Work out the finished part from the listing and answer in its coordinate system (mm). Face numbers are marked on the shaded views. A direction names the side the tool comes from. Give positions to 0.01 mm unless a question says otherwise; leave off trailing zeros. Write each loop counter-clockwise with the first axis right and the second up, starting at its lowest first coordinate (ties: lowest second). Pieces come first, ordered by that corner, then holes. Notation, with made-up numbers: (-24.75, 26) - (-9.75, 26) arc R23 ccw to (-9.75, 36) - close; hole circle Ø10 at (13, 31.25). An arc over 180 degrees is marked (long way). Write item = value, one per line.
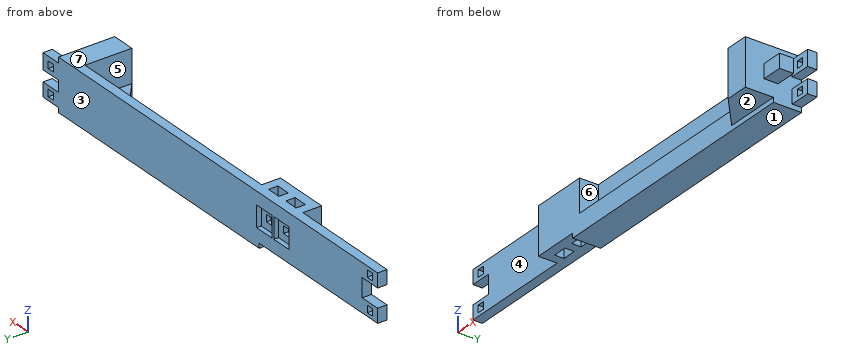
from build123d import *

# Parameters (mm, degrees)
SKETCH2_W           = 194.96
SKETCH2_H           = 6
BOSS_EXTRUDE1_DEPTH = 4
SKETCH3_W           = 176.96
SKETCH3_H           = 4
BOSS_EXTRUDE2_DEPTH = 14
SKETCH4_W           = 6
SKETCH4_H           = 4
BOSS_EXTRUDE3_DEPTH = 9
SKETCH5_W           = 6.8
SKETCH5_H           = 4
BOSS_EXTRUDE4_DEPTH = 9
CUT_EXTRUDE1_REACH  = 197.503
SKETCH6_W           = 3
SKETCH6_H           = 3
SKETCH7_W           = 10
SKETCH7_H           = 20
BOSS_EXTRUDE5_DEPTH = 20
SKETCH8_W           = 136.96
SKETCH8_H           = 6
BOSS_EXTRUDE6_DEPTH = 8
CHAMFER1_SIZE2      = 14.301043111
CHAMFER1_SIZE       = 12
BOSS_EXTRUDE7_DEPTH = 14
CUT_EXTRUDE2_REACH  = 199.001
SKETCH10_W          = 6
SKETCH10_H          = 4
CUT_EXTRUDE3_REACH  = 198.93
SKETCH11_W          = 3
SKETCH11_H          = 3
SKETCH12_W          = 116.96
SKETCH12_H          = 12
BOSS_EXTRUDE8_DEPTH = 2
SKETCH13_W          = 6
SKETCH13_H          = 6
BOSS_EXTRUDE9_DEPTH = 9
SKETCH14_W          = 9
SKETCH14_H          = 9
CUT_EXTRUDE4_DEPTH  = 2


with BuildPart() as part:
    # Sketch2 → Boss-Extrude1 (new body)
    with BuildSketch(Plane(origin=(0, 0, 0), x_dir=(1, 0, 0), z_dir=(0, 1, 0))):
        with Locations((97.48, 3)):
            Rectangle(SKETCH2_W, SKETCH2_H)
    extrude(amount=BOSS_EXTRUDE1_DEPTH)

    # Sketch3 → Boss-Extrude2 (add)
    with BuildSketch(Plane(origin=(0, 0, 0), x_dir=(-1, 0, 0), z_dir=(0, 0, -1))):
        with Locations((-97.48, 2)):
            Rectangle(SKETCH3_W, SKETCH3_H)
    extrude(amount=-BOSS_EXTRUDE2_DEPTH)

    # Sketch4 → Boss-Extrude3 (add)
    with BuildSketch(Plane.ZY.offset(-9)):
        with Locations((11, 2)):
            Rectangle(SKETCH4_W, SKETCH4_H)
    extrude(amount=BOSS_EXTRUDE3_DEPTH)

    # Sketch5 → Boss-Extrude4 (add)
    with BuildSketch(Plane(origin=(185.96, 0, 0), x_dir=(0, 0, -1), z_dir=(1, 0, 0))):
        with Locations((-8.2, 2)):
            Rectangle(SKETCH5_W, SKETCH5_H)
    extrude(amount=BOSS_EXTRUDE4_DEPTH)

    # Sketch6 → Cut-Extrude1 (cut, up to next)
    with BuildSketch(Plane(origin=(0, 4, 0), x_dir=(1, 0, 0), z_dir=(0, 1, 0)), mode=Mode.PRIVATE) as cut_extrude1_sk1:
        with Locations((4.5, 3)):
            Rectangle(SKETCH6_W, SKETCH6_H)
    cut_extrude1_tool1 = extrude(cut_extrude1_sk1.sketch, amount=-CUT_EXTRUDE1_REACH, mode=Mode.PRIVATE) & part.part
    # Sketch6 → Cut-Extrude1 (cut, up to next)
    with BuildSketch(Plane(origin=(0, 4, 0), x_dir=(1, 0, 0), z_dir=(0, 1, 0)), mode=Mode.PRIVATE) as cut_extrude1_sk2:
        with Locations((4.5, -11)):
            Rectangle(SKETCH6_W, SKETCH6_H)
    cut_extrude1_tool2 = extrude(cut_extrude1_sk2.sketch, amount=-CUT_EXTRUDE1_REACH, mode=Mode.PRIVATE) & part.part
    # Sketch6 → Cut-Extrude1 (cut, up to next)
    with BuildSketch(Plane(origin=(0, 4, 0), x_dir=(1, 0, 0), z_dir=(0, 1, 0)), mode=Mode.PRIVATE) as cut_extrude1_sk3:
        with Locations((190.46, 3)):
            Rectangle(SKETCH6_W, SKETCH6_H)
    cut_extrude1_tool3 = extrude(cut_extrude1_sk3.sketch, amount=-CUT_EXTRUDE1_REACH, mode=Mode.PRIVATE) & part.part
    # Sketch6 → Cut-Extrude1 (cut, up to next)
    with BuildSketch(Plane(origin=(0, 4, 0), x_dir=(1, 0, 0), z_dir=(0, 1, 0)), mode=Mode.PRIVATE) as cut_extrude1_sk4:
        with Locations((190.46, -8.2)):
            Rectangle(SKETCH6_W, SKETCH6_H)
    cut_extrude1_tool4 = extrude(cut_extrude1_sk4.sketch, amount=-CUT_EXTRUDE1_REACH, mode=Mode.PRIVATE) & part.part
    add(cut_extrude1_tool1.solids().sort_by_distance((4.5, 4, -3))[0], mode=Mode.SUBTRACT)
    add(cut_extrude1_tool2.solids().sort_by_distance((4.5, 4, 11))[0], mode=Mode.SUBTRACT)
    add(cut_extrude1_tool3.solids().sort_by_distance((190.46, 4, -3))[0], mode=Mode.SUBTRACT)
    add(cut_extrude1_tool4.solids().sort_by_distance((190.46, 4, 8.2))[0], mode=Mode.SUBTRACT)

    # Sketch7 → Boss-Extrude5 (add)
    with BuildSketch(Plane.XZ):
        with Locations((180.96, 4)):
            Rectangle(SKETCH7_W, SKETCH7_H)
    extrude(amount=BOSS_EXTRUDE5_DEPTH)

    # Sketch8 → Boss-Extrude6 (add)
    with BuildSketch(Plane.XZ):
        with Locations((117.48, -3)):
            Rectangle(SKETCH8_W, SKETCH8_H)
    extrude(amount=BOSS_EXTRUDE6_DEPTH)

    # Chamfer1
    chamfer1_edges = [part.edges().sort_by_distance(p)[0] for p in [
        (175.96, -8, -3),
    ]]
    chamfer1_side = [part.faces().sort_by_distance(p)[0] for p in [
        (175.96, -8.24, -3),
    ]]
    chamfer(chamfer1_edges, length=CHAMFER1_SIZE - 0.0001, length2=CHAMFER1_SIZE2 - 0.0001, reference=chamfer1_side[0])  # a hair under: the kernel refuses the full size

    # Sketch9 → Boss-Extrude7 (add)
    with BuildSketch(Plane.XY):
        Polygon((49, -8), (55, -8), (61, -8), (73, -8), (73, 0), (61, 0), (55, 0), (49, 0), align=None)
    extrude(amount=BOSS_EXTRUDE7_DEPTH)

    # Sketch10 → Cut-Extrude2 (cut, up to next)
    with BuildSketch(Plane.XY.offset(14), mode=Mode.PRIVATE) as cut_extrude2_sk1:
        with Locations((56, -2)):
            Rectangle(SKETCH10_W, SKETCH10_H)
    cut_extrude2_tool1 = extrude(cut_extrude2_sk1.sketch, amount=-CUT_EXTRUDE2_REACH, mode=Mode.PRIVATE) & part.part
    # Sketch10 → Cut-Extrude2 (cut, up to next)
    with BuildSketch(Plane.XY.offset(14), mode=Mode.PRIVATE) as cut_extrude2_sk2:
        with Locations((66, -2)):
            Rectangle(SKETCH10_W, SKETCH10_H)
    cut_extrude2_tool2 = extrude(cut_extrude2_sk2.sketch, amount=-CUT_EXTRUDE2_REACH, mode=Mode.PRIVATE) & part.part
    add(cut_extrude2_tool1.solids().sort_by_distance((56, -2, 14))[0], mode=Mode.SUBTRACT)
    add(cut_extrude2_tool2.solids().sort_by_distance((66, -2, 14))[0], mode=Mode.SUBTRACT)

    # Sketch11 → Cut-Extrude3 (cut, up to next)
    with BuildSketch(Plane(origin=(0, 4, 0), x_dir=(1, 0, 0), z_dir=(0, 1, 0)), mode=Mode.PRIVATE) as cut_extrude3_sk1:
        with Locations((56, -4)):
            Rectangle(SKETCH11_W, SKETCH11_H)
    cut_extrude3_tool1 = extrude(cut_extrude3_sk1.sketch, amount=-CUT_EXTRUDE3_REACH, mode=Mode.PRIVATE) & part.part
    # Sketch11 → Cut-Extrude3 (cut, up to next)
    with BuildSketch(Plane(origin=(0, 4, 0), x_dir=(1, 0, 0), z_dir=(0, 1, 0)), mode=Mode.PRIVATE) as cut_extrude3_sk2:
        with Locations((66, -4)):
            Rectangle(SKETCH11_W, SKETCH11_H)
    cut_extrude3_tool2 = extrude(cut_extrude3_sk2.sketch, amount=-CUT_EXTRUDE3_REACH, mode=Mode.PRIVATE) & part.part
    add(cut_extrude3_tool1.solids().sort_by_distance((56, 4, 4))[0], mode=Mode.SUBTRACT)
    add(cut_extrude3_tool2.solids().sort_by_distance((66, 4, 4))[0], mode=Mode.SUBTRACT)

    # Sketch12 → Boss-Extrude8 (add)
    with BuildSketch(Plane(origin=(0, 0, -6), x_dir=(-1, 0, 0), z_dir=(0, 0, -1))):
        with Locations((-127.48, -2)):
            Rectangle(SKETCH12_W, SKETCH12_H)
    extrude(amount=BOSS_EXTRUDE8_DEPTH)

    # Sketch13 → Boss-Extrude9 (add)
    with BuildSketch(Plane(origin=(185.96, 0, 0), x_dir=(0, 0, -1), z_dir=(1, 0, 0))):
        with Locations((-3, -9)):
            Rectangle(SKETCH13_W, SKETCH13_H)
    extrude(amount=BOSS_EXTRUDE9_DEPTH)

    # Sketch14 → Cut-Extrude4 (cut)
    with BuildSketch(Plane(origin=(0, 4, 0), x_dir=(1, 0, 0), z_dir=(0, 1, 0))):
        with Locations((66, -4)):
            Rectangle(SKETCH14_W, SKETCH14_H)
        with Locations((56, -4)):
            Rectangle(SKETCH14_W, SKETCH14_H)
    extrude(amount=-CUT_EXTRUDE4_DEPTH, mode=Mode.SUBTRACT)


solid = part.part
1. Find section C-C, the plane x = 18.5. Give the vertices of the cut face in (y, z).
Solution:
outline = (0, -6) - (4, -6) - (4, 14) - (0, 14) - close
2. Find section A-A, the plane x = 138.5. Give the vertices of the cut face in (y, z), then the cut area to 3 significant figures.
Solution:
outline = (-8, -8) - (4, -8) - (4, 14) - (0, 14) - (0, 0) - (-8, 0) - close
area = 152 mm^2
3. Given pin 1 (1 mm diameter, centred on y = 0.5, z = 3.5, fed in from +X); pin 2 (2 mm diameter, centred on x = 157.5, y = -6.5, fed in from +Z); pin 3 (0.9 mm diameter, centred on x = 4.5, y = 1.5, fed in from -Z), each flat-ended and moving along its own axis, determine where each tip first touches the part or whether it passes through.
Solution:
pin_1 = 185.96
pin_2 = 0
pin_3 = -6
4. For a pull along X with two mould halves and no side action, classify the marked faces 6 and 7 as pulls with the +X half, pulls with the -X half, needs draft (parallel to the pull), parting line crosses it, or undercut.
Solution:
face_6 = undercut
face_7 = needs draft
5. Find section B-B, the plane y = -14.5. Give the vertices of the cut face in (x, z), then the cut area to 3 significant figures.
Solution:
outline = (169.41, -6) - (185.96, -6) - (185.96, 14) - (175.96, 14) - (175.96, 0) - (169.41, 0) - close
area = 239 mm^2
6. Straight lines are drawn through the part: line 1 (X direction, y = 1.25, z = 2.75); line 2 (X direction, y = -0.75, z = -3.5); line 3 (X direction, y = -5, z = 8.75). For each, find the intervals that lie inside material, in ascending order.
Solution:
line_1 = 9 to 54.5, 57.5 to 64.5, 67.5 to 185.96
line_2 = 49 to 53, 59 to 63, 69 to 185.96
line_3 = 49 to 73, 175.96 to 185.96
7. A tool of negligible diameter and unlimited length cuts with its end or side. For the marked faces 1, 2, 3, 4 and 5, from which of +Z, -Z, +X, -X, +Y, -Y can it reach the whole face along a straight path? Write none if from no direction.
Solution:
face_1 = -Z, +X, -X, +Y, -Y
face_2 = -Z, +X, -X, -Y
face_3 = +Z, -Z, +X, -X, +Y
face_4 = +Z, -Z, -X, -Y
face_5 = +Z, -Y
